from build123d import *

# Parameters (mm, degrees)
SALIENTE_EXTRUIR3_DEPTH      = 96.52
SALIENTE_EXTRUIR3_DEPTH_BACK = 152.589992
CROQUIS3_R                   = 74.93
SALIENTE_EXTRUIR4_REACH      = 228.619
CROQUIS4_R                   = 74.93
CROQUIS5_R                   = 78.74
SALIENTE_EXTRUIR5_DEPTH      = 5.08
CROQUIS6_R                   = 81.28
SALIENTE_EXTRUIR6_DEPTH      = 5.08
REDONDEO1_R                  = 2.54
CHAFL_N1_SIZE                = 2.54


# Some blends are built 0.0001 mm under size
with BuildPart() as part:
    # Croquis3 → Saliente-Extruir3 (new, two sides: drawn at the far end of the back side and taken through both)
    with BuildSketch(Plane(origin=(0, 0, 0), x_dir=(0, 0, -1), z_dir=(1, 0, 0)).offset(-SALIENTE_EXTRUIR3_DEPTH_BACK)):
        Circle(CROQUIS3_R)
    extrude(amount=SALIENTE_EXTRUIR3_DEPTH + SALIENTE_EXTRUIR3_DEPTH_BACK)

    # Croquis4 → Saliente-Extruir4 (add, up to next)
    with BuildSketch(Plane(origin=(0, 74.93, 0), x_dir=(1, 0, 0), z_dir=(0, 1, 0)), mode=Mode.PRIVATE) as saliente_extruir4_sk1:
        Circle(CROQUIS4_R)
    saliente_extruir4_tool1 = extrude(saliente_extruir4_sk1.sketch, amount=-SALIENTE_EXTRUIR4_REACH, mode=Mode.PRIVATE) - part.part
    add(saliente_extruir4_tool1.solids().sort_by_distance((0, 74.93, 0))[0])
    add(saliente_extruir4_tool1.solids().sort_by_distance((0, 74.93, 0))[1])

    # Croquis5 → Saliente-Extruir5 (add)
    with BuildSketch(Plane.ZY.offset(152.589992)):
        Circle(CROQUIS5_R)
    extrude(amount=SALIENTE_EXTRUIR5_DEPTH)

    # Croquis6 → Saliente-Extruir6 (add)
    with BuildSketch(Plane.ZY.offset(157.669992)):
        Circle(CROQUIS6_R)
    extrude(amount=SALIENTE_EXTRUIR6_DEPTH)

    # Redondeo1
    redondeo1_edges = [part.edges().sort_by_distance(p)[0] for p in [
        (-157.669992, 0, -81.28),
    ]]
    fillet(redondeo1_edges, radius=REDONDEO1_R - 0.0001)  # a hair under: the kernel refuses the full size

    # Chaflán1
    # the kernel refuses this chamfer: 2.54 mm, written as the material it takes off along each edge
    with BuildSketch(Plane(origin=(96.52, 0, 0), x_dir=(0, 0, -1), z_dir=(0, -1, 0))) as chafl_n1_piece_1:
        Polygon((74.93, -CHAFL_N1_SIZE), (74.93 - CHAFL_N1_SIZE, 0), (74.93, 0), align=None)
    revolve(axis=Axis((96.52, 0, 0), (1, 0, 0)), mode=Mode.SUBTRACT)


solid = part.part
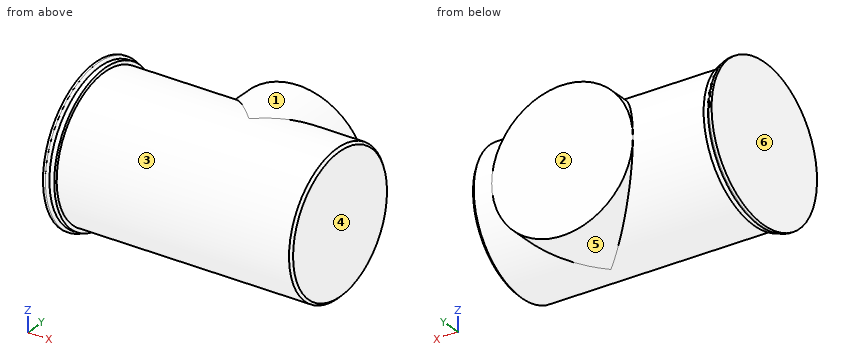
Work out the finished part from the listing and answer in its coordinate system (mm). Face numbers are marked on the shaded views. A direction names the side the tool comes from. Round coordinates to 2 decimals unless told otherwise and drop trailing zeros. Write each loop counter-clockwise with the first axis right and the second up, starting at its lowest first coordinate (ties: lowest second). Pieces come first, ordered by that corner, then holes.
1) A cutting plane is placed at A-A (x = -116). Give the vertices of the cut face in (y, z).
2) Given pin 1 Ø10 at (x, z) = (49.5, 18.5) entering from +Y; pin 2 Ø1 at (x, y) = (-42.5, 60.5) entering from -Z; pin 3 Ø4 at (x, z) = (-40.5, -52) entering from -Y, each flat-ended and moving along its own axis, determine where each tip first touches the part or whether it passes through.
3) A cutting plane is placed at B-B (x = 0). Give the vertices of the cut face in (y, z).
4) A tool of negligible diameter and unlimited length cuts with its end or side. For the marked faces 1 and 2, from which of +Z, -Z, +X, -X, +Y, -Y can it reach the whole face along a straight path? Write none if from no direction.
5) Straight lines are drawn through the part: line 1 (Y direction, x = -60, z = -2); line 2 (Y direction, x = -151.5, z = -56); line 3 (Z direction, x = 67, y = -60.5). For each, find the intervals that lie inside material, in ascending order.
6) The mould has two halves that part along X. Classify the marked faces 3, 4, 5 and 6: pulls with the +X half, pulls with the -X half, needs draft (parallel to the pull), parting line crosses it, or undercut.
7) A cutting plane is placed at C-C (x = 32). Give the vertices of the cut face in (y, z).
Completed:
1. outline: circle Ø149.86 at (0, 0)
2. pin 1: stops at y = 74.93
2. pin 2: stops at z = -62.05
2. pin 3: stops at y = -55.81
3. outline: (0, -74.93) - (74.93, -74.93) - (74.93, 74.93) - (0, 74.93) arc R74.93 ccw to start
4. face 1: +Z, +Y
4. face 2: +Z, -Z, +X, +Y
5. line 1: y = -74.9 to 74.93
5. line 2: y = -49.78 to 49.78
5. line 3: z = -44.21 to 44.21
6. face 3: undercut
6. face 4: pulls with the +X half
6. face 5: undercut
6. face 6: pulls with the -X half
7. outline: (32, -67.75) - (74.93, -67.75) - (74.93, 67.75) - (32, 67.75) arc R74.93 ccw (long way) to start
